Verification items for the finished model (mm, model axes). Face numbers are marked on the shaded views. Round coordinates to 2 decimals unless told otherwise and drop trailing zeros. Write each loop counter-clockwise with the first axis right and the second up, starting at its lowest first coordinate (ties: lowest second). Pieces come first, ordered by that corner, then holes. Notation, with made-up numbers: M -13,49.5 L 11,49.5 A26 ccw 11,80.5 Z; hole C -14,61 d6. An arc over 180 degrees is marked long. Use a Markdown table: item, result. Add a question column.
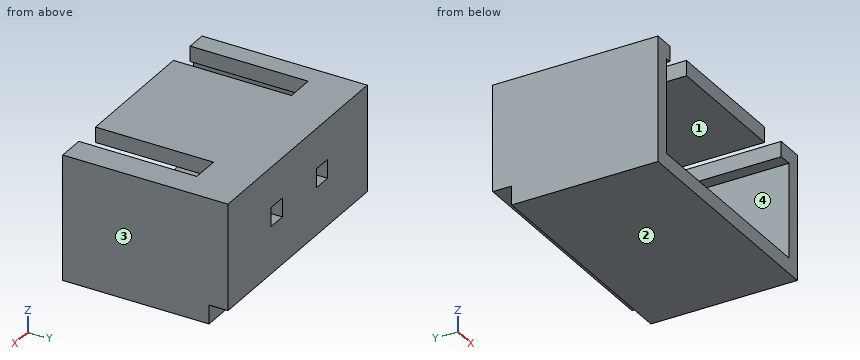
from build123d import *

# Parameters (mm, degrees)
SKETCH1_W           = 10
SKETCH1_H           = 5.3
BOSS_EXTRUDE1_DEPTH = 7
SKETCH3_W           = 8.8
SKETCH3_H           = 4
CUT_EXTRUDE1_DEPTH  = 5
SKETCH4_W           = 1.2
SKETCH4_H           = 5
CUT_EXTRUDE2_DEPTH  = 4
SKETCH5_W           = 10
SKETCH5_H           = 0.8
CUT_EXTRUDE3_DEPTH  = 0.8
SKETCH6_W           = 0.8
SKETCH6_H           = 0.8
CUT_EXTRUDE4_DEPTH  = 10
SKETCH7_W           = 8.8
SKETCH7_H           = 1
CUT_EXTRUDE5_DEPTH  = 0.3


with BuildPart() as part:
    # Sketch1 → Boss-Extrude1 (new body)
    with BuildSketch(Plane(origin=(0, 0, 0), x_dir=(1, 0, 0), z_dir=(0, 1, 0))):
        Rectangle(SKETCH1_W, SKETCH1_H)
    extrude(amount=BOSS_EXTRUDE1_DEPTH)

    # Sketch3 → Cut-Extrude1 (cut)
    with BuildSketch(Plane.XZ):
        Rectangle(SKETCH3_W, SKETCH3_H)
    extrude(amount=-CUT_EXTRUDE1_DEPTH, mode=Mode.SUBTRACT)

    # Sketch4 → Cut-Extrude2 (cut)
    with BuildSketch(Plane.XY.offset(2.65)):
        with Locations((-3.55, 2.5)):
            Rectangle(SKETCH4_W, SKETCH4_H)
        with Locations((3.25, 2.5)):
            Rectangle(SKETCH4_W, SKETCH4_H)
    extrude(amount=-CUT_EXTRUDE2_DEPTH, mode=Mode.SUBTRACT)

    # Sketch5 → Cut-Extrude3 (cut)
    with BuildSketch(Plane(origin=(0, 7, 0), x_dir=(1, 0, 0), z_dir=(0, 1, 0))):
        with Locations((0, 2.25)):
            Rectangle(SKETCH5_W, SKETCH5_H)
    extrude(amount=-CUT_EXTRUDE3_DEPTH, mode=Mode.SUBTRACT)

    # Sketch6 → Cut-Extrude4 (cut)
    with BuildSketch(Plane(origin=(0, 7, 0), x_dir=(1, 0, 0), z_dir=(0, 1, 0))):
        with Locations((1.5, -0.55)):
            Rectangle(SKETCH6_W, SKETCH6_H)
        with Locations((-1.75, -0.55)):
            Rectangle(SKETCH6_W, SKETCH6_H)
    extrude(amount=-CUT_EXTRUDE4_DEPTH, mode=Mode.SUBTRACT)

    # Sketch7 → Cut-Extrude5 (cut)
    with BuildSketch(Plane.XZ.offset(-5)):
        with Locations((0, -1.5)):
            Rectangle(SKETCH7_W, SKETCH7_H)
    extrude(amount=-CUT_EXTRUDE5_DEPTH, mode=Mode.SUBTRACT)


solid = part.part
1. Scan lines: line 1 along X through (y, z) = (3.75, 1.1); line 2 along Z through (x, y) = (1.75, 5.5); line 3 along Z through (x, y) = (-1, 3.75). Record each from-to range of solid material in increasing order. Write a range as from..to.
2. Cross-section at A-A on x = -2. Enter the section's corners in (y, z).
3. Cross-section at D-D on z = -1.5. Enter the section's corners in (x, y).
4. Release check for a two-part mould opening along X. For the marked faces 1, 2, 3 and 4 record: +X half, -X half, draft (parallel to the pull), parting line (faces both ways), or undercut.
5. Cross-section at C-C on y = 6. Enter the section's corners in (x, z).
6. Cross-section at B-B on y = 3.5. Enter the section's corners in (x, z).
Answer:
| question | item | result |
|---|---|---|
| 1 | line 1 | x = -5..-4.4, 4.4..5 |
| 1 | line 2 | z = -2.65..0.15, 0.95..2.65 |
| 1 | line 3 | z = -2.65..-2, 2..2.65 |
| 2 | outline | M 0,-2.65 L 6.2,-2.65 L 6.2,-1.85 L 7,-1.85 L 7,0.15 L 5,0.15 L 5,-1 L 5.3,-1 L 5.3,-2 L 0,-2 Z; M 0,2 L 5,2 L 5,0.95 L 7,0.95 L 7,2.65 L 0,2.65 Z |
| 3 | outline | M -5,0 L -4.4,0 L -4.4,5.3 L 4.4,5.3 L 4.4,0 L 5,0 L 5,7 L -5,7 Z |
| 4 | face 1 | undercut |
| 4 | face 2 | draft |
| 4 | face 3 | +X half |
| 4 | face 4 | undercut |
| 5 | outline | M -5,-2.65 L 5,-2.65 L 5,2.65 L -5,2.65 Z; hole M -2.15,0.15 L -1.35,0.15 L -1.35,0.95 L -2.15,0.95 Z; hole M 1.1,0.15 L 1.9,0.15 L 1.9,0.95 L 1.1,0.95 Z |
| 6 | outline | M -5,-2.65 L 5,-2.65 L 5,2.65 L 3.85,2.65 L 3.85,2 L 4.4,2 L 4.4,-2 L -4.4,-2 L -4.4,2 L -4.15,2 L -4.15,2.65 L -5,2.65 Z; M -2.95,2 L 2.65,2 L 2.65,2.65 L -2.95,2.65 Z |
